Autodesk Inventor part; units mm, degrees
ref_plane "YZ Plane" through (0, 0, 0) normal (1, 0, 0) x (0, 1, 0)
ref_plane "XZ Plane" through (0, 0, 0) normal (0, 1, 0) x (-1, 0, 0)
ref_plane "XY Plane" through (0, 0, 0) normal (0, 0, 1) x (1, 0, 0)
sketch "Sketch1" plane through (0, 0, 0) normal (0, 0, 1) x (1, 0, 0)
  line L0 (0, 0) -> (525.78, 0)
  line L1 (0, 0) -> (0, 101.6)
  line L2 (0, 101.6) -> (262.89, 253.3796)
  line L3 (262.89, 253.3796) -> (525.78, 101.6)
  line L4 (525.78, 101.6) -> (525.78, 0)
  line L5 (262.89, 246.0473) -> (6.35, 97.9338)
  line L6 (6.35, 97.9338) -> (6.35, 6.35)
  line L7 (6.35, 6.35) -> (519.43, 6.35)
  line L8 (519.43, 6.35) -> (519.43, 97.9338)
  line L9 (519.43, 97.9338) -> (262.89, 246.0473)
  point P0 (262.89, 0)
  dimension "d0" = 525.78
  dimension "d1" = 101.6
  dimension "d2" = 120
  dimension "d3" = 6.35
extrude "Extrusion1" add sketch "Sketch1" along normal blind 355.6
sketch "Sketch2" plane through (0, 0, 355.6) normal (0, 0, 1) x (1, 0, 0)
  line L0 (262.89, 246.0473) -> (519.43, 97.9338)
  line L1 (519.43, 97.9338) -> (519.43, 6.35)
  line L2 (519.43, 6.35) -> (6.35, 6.35)
  line L3 (6.35, 6.35) -> (6.35, 97.9338)
  line L4 (6.35, 97.9338) -> (262.89, 246.0473)
  line L5 (0, 0) -> (525.78, 0)
  line L6 (525.78, 0) -> (525.78, 101.6)
  line L7 (525.78, 101.6) -> (262.89, 253.3796)
  line L8 (262.89, 253.3796) -> (0, 101.6)
  line L9 (0, 101.6) -> (0, 0)
  circle A0 centre (262.89, 121.3796) radius 60
  dimension "d6" = 120
  dimension "d7" = 132
extrude "Extrusion2" add sketch "Sketch2" along normal blind 6.35 contours L0 L1 L2 L3 L4 | L9 L8 L7 L6 L5
sketch "Sketch3" plane through (0, 0, 0) normal (0, -1, 0) x (1, 0, 0)
  line L0 (0, 0) -> (525.78, 0) construction
  line L1 (525.78, 0) -> (525.78, 88.9)
  line L2 (525.78, 88.9) -> (0, 88.9) construction
  line L3 (0, 88.9) -> (0, 0) construction
  line L4 (86.36, 21.95) -> (86.36, 66.95) construction
  circle A0 centre (86.36, 44.45) radius 2.3812
  circle A1 centre (86.36, 21.95) radius 2.3812
  circle A2 centre (86.36, 66.95) radius 2.3812
  line L5 (146.36, 49.45) -> (146.36, 29.45) construction
  line L6 (156.36, 66.95) -> (156.36, 21.95) construction
  line L7 (146.36, 29.45) -> (166.36, 29.45) construction
  line L8 (166.36, 49.45) -> (146.36, 49.45) construction
  line L9 (86.36, 66.95) -> (226.36, 66.95) construction
  line L10 (226.36, 21.95) -> (86.36, 21.95) construction
  line L11 (86.36, 44.45) -> (226.36, 44.45) construction
  line L12 (166.36, 29.45) -> (166.36, 49.45) construction
  line L13 (226.36, 66.95) -> (226.36, 21.95) construction
  circle A3 centre (226.36, 66.95) radius 2.3813
  circle A4 centre (226.36, 44.45) radius 2.3813
  circle A5 centre (226.36, 21.95) radius 2.3813
  circle A6 centre (156.36, 39.45) radius 10
  line L14 (0, 0) -> (0, 361.95)
  line L15 (525.78, 0) -> (525.78, 361.95)
  line L16 (0, 0) -> (525.78, 0)
  point P0 (0, 44.45)
  point P1 (146.36, 39.45)
  point P2 (166.36, 39.45)
  point P3 (262.89, 0)
  dimension "d10" = 45
  dimension "d11" = 140
  dimension "d12" = 4.7625
  dimension "d13" = 4.7625
  dimension "d14" = 4.7625
  dimension "d15" = 4.7625
  dimension "d16" = 4.7625
  dimension "d17" = 4.7625
  dimension "d18" = 60
  dimension "d19" = 7.5
  dimension "d20" = 20
  dimension "d21" = 20
  dimension "d22" = 86.36
  dimension "d23" = 88.9
extrude "Extrusion3" cut sketch "Sketch3" against normal blind 6.35
sketch "Sketch4" plane through (0, 0, 0) normal (0, -1, 0) x (1, 0, 0)
  line L0 (71.36, 0) -> (241.36, 0)
  line L1 (241.36, 0) -> (241.36, 85)
  line L2 (241.36, 85) -> (71.36, 85)
  line L3 (71.36, 85) -> (71.36, 0)
  line L4 (0, 0) -> (525.78, 0) construction
  circle A0 centre (156.36, 39.45) radius 10 construction
  point P0 (156.36, 85)
  dimension "d26" = 170
  dimension "d27" = 85
extrude "Extrusion4" cut sketch "Sketch4" against normal blind 6.35
sketch "Sketch5" plane through (0, 0, 361.95) normal (0, -1, 0) x (1, 0, 0)
  line L0 (525.78, -361.95) -> (525.78, 0)
  line L1 (525.78, -361.95) -> (0, -361.95)
  line L2 (0, -361.95) -> (0, -243.4167)
  line L3 (0, -243.4167) -> (525.78, -243.4167)
  line L4 (525.78, -243.4167) -> (525.78, -361.95)
  line L5 (525.78, -243.4167) -> (0, -243.4167)
  line L6 (0, -243.4167) -> (0, -124.8833)
  line L7 (0, -124.8833) -> (525.78, -124.8833)
  line L8 (525.78, -124.8833) -> (525.78, -243.4167)
  line L9 (262.89, 0) -> (0, 0)
  line L10 (525.78, -124.8833) -> (0, -124.8833)
  line L11 (0, -124.8833) -> (0, 0)
  line L12 (0, 0) -> (525.78, 0)
  line L13 (525.78, 0) -> (525.78, -124.8833)
  line L14 (0, -361.95) -> (0, 0)
  point P0 (0, -184.15)
  dimension "d30" = 118.5333
  dimension "d31" = 118.5333
extrude "Extrusion5" cut sketch "Sketch5" against normal through all contours L1 L2 L3 L0 | L7 L11 L9 L12 L0
properties part number "CA01" material "ABS Plastic"
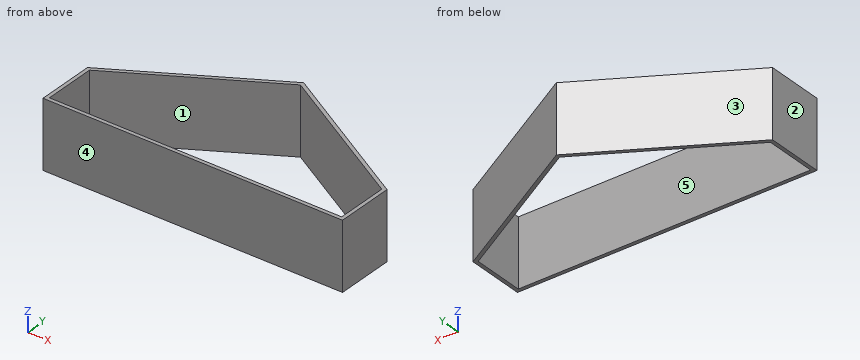
Verification items for the finished model (mm, model axes). Face numbers are marked on the shaded views. A direction names the side the tool comes from. Coordinates: 2 decimals unless noted, no trailing zeros. Loops run counter-clockwise (first coordinate to the right, second up) from the corner with the lowest first, then second, coordinate; pieces in that order, holes last. Notation, with made-up numbers: (53, 48) - (76, 48) arc R4 cw to (76, 54) - close; hole circle Ø3 at (82.25, 52.25). An arc over 180 degrees is marked (long way). Answer as a JSON object with one key per item and string values.
(1) Cross-section at B-B, the plane x = 270. Record the boundary of the cut face in (y, z), then the cut area to 3 significant figures.
Response:
{"outline": "(0, 118.53) - (6.35, 118.53) - (6.35, 237.07) - (0, 237.07) - close; (241.94, 118.53) - (249.27, 118.53) - (249.27, 237.07) - (241.94, 237.07) - close", "area": "1,620 mm²"}
(2) Cross-section at A-A, the plane y = 17. Record the boundary of the cut face in (x, z).
Response:
{"outline": "(0, 118.53) - (6.35, 118.53) - (6.35, 237.07) - (0, 237.07) - close; (519.43, 118.53) - (525.78, 118.53) - (525.78, 237.07) - (519.43, 237.07) - close"}
(3) Scan lines: line 1 along X through (y, z) = (74.5, 141); line 2 along X through (y, z) = (204, 153); line 3 along Y through (x, z) = (432, 164). Record each from-to range of solid material in increasing order.
Response:
{"line 1": "x = 0 to 6.35, 519.43 to 525.78", "line 2": "x = 177.36 to 190.06, 335.72 to 348.42", "line 3": "y = 0 to 6.35, 148.41 to 155.74"}
(4) Cross-section at C-C, the plane z = 171. Record the boundary of the cut face in (x, y).
Response:
{"outline": "(0, 0) - (525.78, 0) - (525.78, 101.6) - (262.89, 253.38) - (0, 101.6) - close; hole (6.35, 6.35) - (519.43, 6.35) - (519.43, 97.93) - (262.89, 246.05) - (6.35, 97.93) - close"}
(5) Access from +Z, -Z, +X, -X, +Y, -Y to the whole of each face (thin tool, end or side, straight path). Record for the marked faces 4 and 5.
Response:
{"face 4": "+Z, -Z, +X, -X, -Y", "face 5": "+Z, -Z"}
(6) Go/stop test with flat-tipped pins: pin 1 Ø8 at (y, z) = (157.5, 132.5) entering from -X; pin 2 Ø4 at (y, z) = (171, 173.5) entering from +X; pin 3 Ø8 at (x, z) = (170, 180) entering from +Y. Record where each tip stops, or that it passes through.
Response:
{"pin 1": "stops at x = 89.89", "pin 2": "stops at x = 409.04", "pin 3": "stops at y = 202.06"}
(7) Mould release check, pull along Y, two halves, no side actions. Record for the marked faces 1, 2 and 3: pulls with the +Y half, pulls with the -Y half, needs draft (parallel to the pull), parting line crosses it, or undercut.
Response:
{"face 1": "undercut", "face 2": "needs draft", "face 3": "pulls with the +Y half"}
